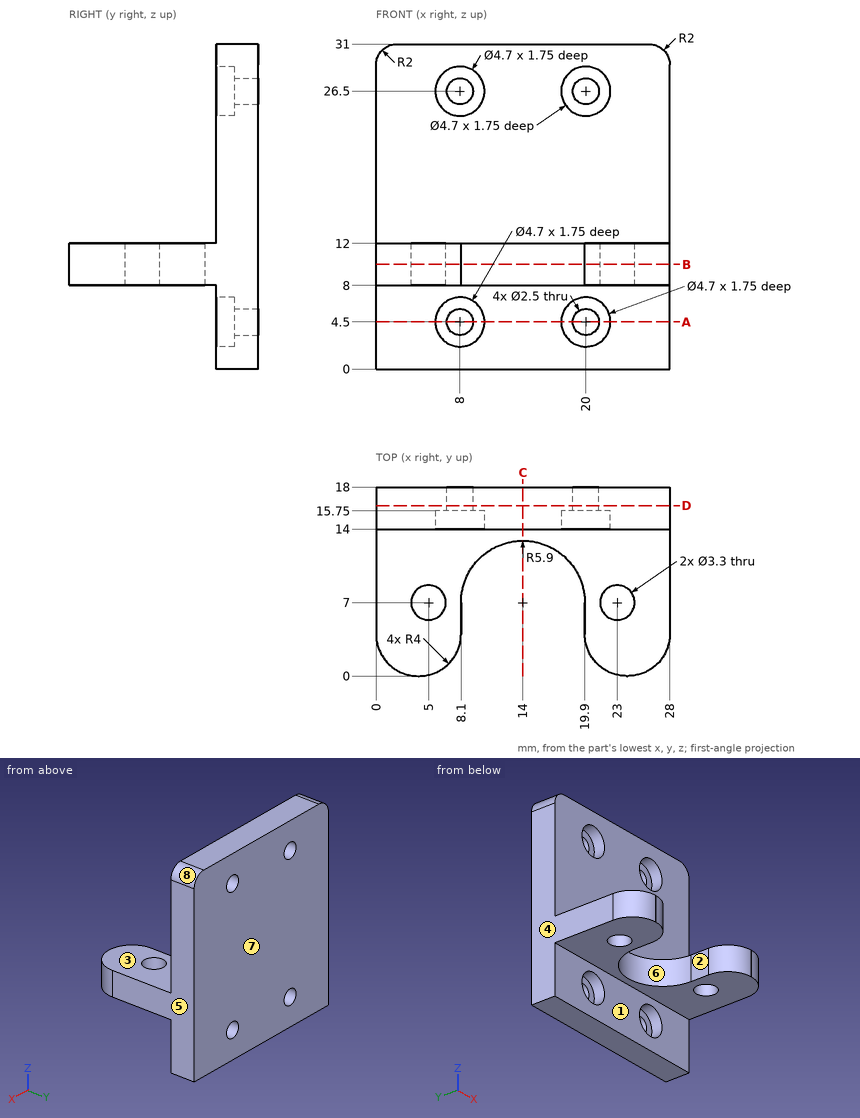
Here's the drawing with two shaded views (mm, measured from the low corner). I have some questions. A direction names the side the tool comes from. Coordinates: 2 decimals unless noted, no trailing zeros. Write each loop counter-clockwise with the first axis right and the second up, starting at its lowest first coordinate (ties: lowest second). Pieces come first, ordered by that corner, then holes. Notation, with made-up numbers: M 41,75.5 L 77,75.5 A6 ccw 77,82.5 Z; hole C 21.25,64.25 d10. An arc over 180 degrees is marked long. Write item = value, one per line. Start each with the question number.
Q1. If we section it at B-B, the plane z = 10: Write out the boundary of the cut face in (x, y), then the cut area to 3 significant figures.
Q2. Thinking about a two-plate mould opening in X: for the marked faces 6, 7 and 8, which applies, released by +X, released by -X, zero draft, split by the parting line, or undercut?
Q3. If we section it at C-C, the plane x = 14: Write out the boundary of the cut face in (y, z), then the cut area to 3 significant figures.
Q4. On a 3-axis mill with a long thin cutter (end or side, diameter ignored), from which of +Z, -Z, +X, -X, +Y, -Y can I reach the whole of each face in a straight line? I mean the marked faces 1, 2, 3, 4 and 5. Say none if no direction works.
Q5. If we section it at D-D, the plane y = 16.25: Write out the boundary of the cut face in (x, z), then the cut area to 3 significant figures.
Q6. If we section it at A-A, the plane z = 4.5: Write out the boundary of the cut face in (x, y), then the cut area to 3 significant figures.
Q7. I'm going to push flat-ended pins straight in: pin 1 (1.5 mm diameter, centred on x = 20, z = 26.5, fed in from +Y); pin 2 (2.5 mm diameter, centred on x = 20, z = 26, fed in from -Y); pin 3 (5 mm diameter, centred on x = 8, z = 26.5, fed in from -Y); pin 4 (5.5 mm diameter, centred on x = 23, y = 7, fed in from +Z). Where does each tip first touch, or does it pass through?
Q8. If I drill on L1, parallel to X at y = 7, z = 9.7; L2, parallel to Z at x = 8, y = 15.2; L3, parallel to Z at x = 8, y = 16.3, over which ranges is the centre line in solid material (lowest first)? Write a range as [from, to].
Check sheet entries:
q1.outline = M 0,4 A4 ccw 4,0 L 4.1,0 A4 ccw 8.1,4 L 8.1,7 A5.9 cw 19.9,7 L 19.9,4 A4 ccw 23.9,0 L 24,0 A4 ccw 28,4 L 28,18 L 0,18 Z; hole C 5,7 d3.3; hole C 23,7 d3.3
q1.area = 336 mm²
q2.face_6 = undercut
q2.face_7 = zero draft
q2.face_8 = released by +X
q3.outline = M 12.9,8 L 14,8 L 14,0 L 18,0 L 18,31 L 14,31 L 14,12 L 12.9,12 Z
q3.area = 128 mm²
q4.face_1 = -Z, +X, -X, -Y
q4.face_2 = +Z, -Z, -Y
q4.face_3 = +Z, +X, -X, -Y
q4.face_4 = +Z, -Z, -X, +Y, -Y
q4.face_5 = +Z, -Z, +X, +Y, -Y
q5.outline = M 0,0 L 28,0 L 28,29 A2 ccw 26,31 L 2,31 A2 ccw 0,29 Z; hole C 8,4.5 d2.5; hole C 8,26.5 d2.5; hole C 20,4.5 d2.5; hole C 20,26.5 d2.5
q5.area = 847 mm²
q6.outline = M 0,14 L 5.65,14 L 5.65,15.75 L 6.75,15.75 L 6.75,18 L 0,18 Z; M 9.25,15.75 L 10.35,15.75 L 10.35,14 L 17.65,14 L 17.65,15.75 L 18.75,15.75 L 18.75,18 L 9.25,18 Z; M 21.25,15.75 L 22.35,15.75 L 22.35,14 L 28,14 L 28,18 L 21.25,18 Z
q6.area = 84.3 mm²
q7.pin_1 = through
q7.pin_2 = 15.75
q7.pin_3 = 14
q7.pin_4 = 12
q8.L1 = [0, 3.35], [6.65, 8.1], [19.9, 21.35], [24.65, 28]
q8.L2 = [0, 2.15], [6.85, 24.15], [28.85, 31]
q8.L3 = [0, 3.25], [5.75, 25.25], [27.75, 31]
